```python
from build123d import *

# Parameters (mm, degrees)
F0_R     = 50.8
F1_DEPTH = 1.524


with BuildPart() as f1:
    # F0 (on Front) → F1 (new body)
    with BuildSketch(Plane.XZ):
        Circle(F0_R)
        with BuildLine():
            ThreePointArc((-32.743325, -25.544716), (-41.334156, -4.018132), (-37.050229, 18.76002))
            ThreePointArc((-37.050229, 18.76002), (-23.2074, 23.935861), (-14.817719, 11.769246))
            ThreePointArc((-14.817719, 11.769246), (-18.826709, -1.906553), (-12.157372, -14.500974))
            ThreePointArc((-12.157372, -14.500974), (-18.09988, -28.132282), (-32.743325, -25.544716))
        make_face(mode=Mode.SUBTRACT)
        with BuildLine():
            ThreePointArc((32.743325, -25.544716), (18.588573, -26.668251), (13.248466, -13.511406))
            ThreePointArc((13.248466, -13.511406), (18.876275, -1.328977), (15.01092, 11.521814))
            ThreePointArc((15.01092, 11.521814), (23.259145, 23.579527), (37.050229, 18.76002))
            ThreePointArc((37.050229, 18.76002), (41.334156, -4.018132), (32.743325, -25.544716))
        make_face(mode=Mode.SUBTRACT)
    extrude(amount=F1_DEPTH)


solid = f1.part
```
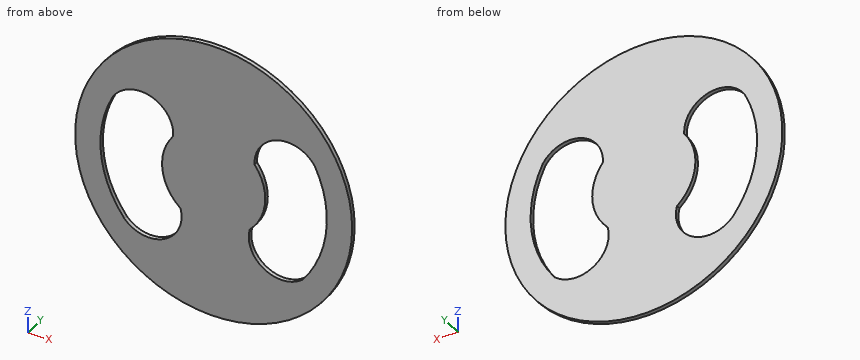
The model under review builds one solid part; all positions refer to its coordinate system, in mm. Round coordinates to 2 decimals unless told otherwise and drop trailing zeros. Order: outer loops, then holes, each group sorted by start corner. A loop starts at its lowest first (then second) coordinate and runs counter-clockwise, first axis right, second up. Notation, with made-up numbers: (9, 23) -> (13, 23) arc R32 cw to (13, 62) -> close; hole circle Ø1 at (11, -28). An arc over 180 degrees is marked (long way). One line per item, written item: value. Start each with the question number.
Q1. Wall thickness on line 1 (X direction, y = -0.4, z = 0.5); line 2 (Z direction, x = 17, y = -0.85); line 3 (X direction, y = -0.15, z = 23): over which ranges is each line inside the solid? List them lowest first.
Q2. Take a section at C-C (y = -0.75). Write out the cut boundary in (x, z), and give its area (3 significant figures).
Q3. Clearance check with a flat-ended pin moving along its axis: pin 1 Ø10 at (x, z) = (39, 12) entering from +Y. State where the tip first meets the part, or that it passes through.
Q4. Take a section at D-D (x = -17). Write out the cut boundary in (y, z), and give its area (3 significant figures).
Q5. Take a section at B-B (x = 26.5). Write out the cut boundary in (y, z), and give its area (3 significant figures).
Q6. Take a section at A-A (z = 0). Write out the cut boundary in (x, y).
Reported:
1. line 1: x = -50.8 to -41.53, -18.92 to 18.92, 41.53 to 50.8
1. line 2: z = -47.87 to -25.5, -8.31 to 8.31, 18.81 to 47.87
1. line 3: x = -45.3 to -32.6, -21.02 to 21.82, 32.2 to 45.3
2. outline: circle Ø101.6 at (0, 0); hole (-37.05, 18.76) arc R41.53 ccw to (-32.74, -25.54) arc R12.01 ccw to (-12.16, -14.5) arc R18.92 cw to (-14.82, 11.77) arc R12.01 ccw to start; hole (13.25, -13.51) arc R12.01 ccw to (32.74, -25.54) arc R41.53 ccw to (37.05, 18.76) arc R12.01 ccw to (15.01, 11.52) arc R18.92 cw to start
2. area: 5,800 mm2
3. pin 1: stops at y = 0
4. outline: (-1.52, -47.87) -> (0, -47.87) -> (0, -27.46) -> (-1.52, -27.46) -> close; (-1.52, -8.31) -> (0, -8.31) -> (0, 8.31) -> (-1.52, 8.31) -> close; (-1.52, 19.41) -> (0, 19.41) -> (0, 47.87) -> (-1.52, 47.87) -> close
4. area: 99.8 mm2
5. outline: (-1.52, -43.34) -> (0, -43.34) -> (0, -28.35) -> (-1.52, -28.35) -> close; (-1.52, 24.17) -> (0, 24.17) -> (0, 43.34) -> (-1.52, 43.34) -> close
5. area: 52.1 mm2
6. outline: (-50.8, -1.52) -> (-41.53, -1.52) -> (-41.53, 0) -> (-50.8, 0) -> close; (-18.92, -1.52) -> (18.92, -1.52) -> (18.92, 0) -> (-18.92, 0) -> close; (41.53, -1.52) -> (50.8, -1.52) -> (50.8, 0) -> (41.53, 0) -> close
